Design review of the part built by this model. Coordinates are the model's own, in mm. Give positions to 0.01 mm unless a question says otherwise; leave off trailing zeros. Loops run counter-clockwise (first coordinate to the right, second up) from the corner with the lowest first, then second, coordinate; pieces in that order, holes last. Notation, with made-up numbers: M -33,-28 L 19,-28 A35 cw 19,10 Z; hole C 11,19.25 d2. An arc over 180 degrees is marked long. Use CSV: the item, a comma, the result in double quotes.
from build123d import *

# Parameters (mm, degrees)
SKETCH_W  = 25
SKETCH_H  = 110
SKETCH_R  = 8.5
PAD_DEPTH = 25


with BuildPart() as part:
    # Sketch → Pad (new body)
    with BuildSketch(Plane.XZ):
        Rectangle(SKETCH_W, SKETCH_H)
        with Locations((0, -30)):
            Circle(SKETCH_R, mode=Mode.SUBTRACT)
        with Locations((0, 5)):
            Circle(SKETCH_R, mode=Mode.SUBTRACT)
    extrude(amount=PAD_DEPTH)


solid = part.part
(1) We need section D-D on x = -6.25. State the section outline as (y, z) points.
A:
outline,"M -25,-55 L 0,-55 L 0,-35.76 L -25,-35.76 Z; M -25,-24.24 L 0,-24.24 L 0,-0.76 L -25,-0.76 Z; M -25,10.76 L 0,10.76 L 0,55 L -25,55 Z"
(2) We need section B-B on z = 5. State the section outline as (x, y) points.
A:
outline,"M -12.5,-25 L -8.5,-25 L -8.5,0 L -12.5,0 Z; M 8.5,-25 L 12.5,-25 L 12.5,0 L 8.5,0 Z"
(3) We need section C-C on y = -8.5. State the section outline as (x, z) points.
A:
outline,"M -12.5,-55 L 12.5,-55 L 12.5,55 L -12.5,55 Z; hole C 0,-30 d17; hole C 0,5 d17"
(4) Wall thickness on line 1 along Z through (x, y) = (0, -8); line 2 along Z through (x, y) = (-7.5, -13); line 3 along X through (y, z) = (-20.5, -26.5): over which ranges is each line inside the solid? List them lowest first. Write a range as [from, to].
A:
line 1,"[-55, -38.5], [-21.5, -3.5], [13.5, 55]"
line 2,"[-55, -34], [-26, 1], [9, 55]"
line 3,"[-12.5, -7.75], [7.75, 12.5]"
(5) The part is to be moulded in two halves that separate along Z. For faces 1 (the flat face through (0, -12, 55)), 2 (the flat face through (-9, -25, 1)), 3 (the cylindrical face through (-1.107, -12.325, 13.428)), say which applies: released by +Z, released by -Z, zero draft, split by the parting line, or undercut.
A:
face 1,"released by +Z"
face 2,"zero draft"
face 3,"undercut"
(6) We need section A-A on x = 0. State the section outline as (y, z) points.
A:
outline,"M -25,-55 L 0,-55 L 0,-38.5 L -25,-38.5 Z; M -25,-21.5 L 0,-21.5 L 0,-3.5 L -25,-3.5 Z; M -25,13.5 L 0,13.5 L 0,55 L -25,55 Z"
